```python
from build123d import *

# Parameters (mm, degrees)
SKETCH2_R           = 26.533992322
BOSS_EXTRUDE1_DEPTH = 5.7658
CHAMFER1_SIZE       = 1.27
SKETCH3_R           = 8.509
CUT_EXTRUDE1_DEPTH  = 5.7658
CHAMFER2_SIZE       = 1.016


with BuildPart() as part:
    # Sketch2 → Boss-Extrude1 (new body)
    with BuildSketch(Plane.XY):
        with Locations(Location((0, 0, 0), (0, 0, 180))):
            Circle(SKETCH2_R)
    extrude(amount=BOSS_EXTRUDE1_DEPTH)

    # Chamfer1
    chamfer1_edges = [part.edges().sort_by_distance(p)[0] for p in [
        (26.533992322, 0, 0),
        (26.533992322, 0, 5.7658),
    ]]
    chamfer(chamfer1_edges, length=CHAMFER1_SIZE)

    # Sketch3 → Cut-Extrude1 (cut)
    with BuildSketch(Plane.XY.offset(5.7658)):
        Circle(SKETCH3_R)
    extrude(amount=-CUT_EXTRUDE1_DEPTH, mode=Mode.SUBTRACT)

    # Chamfer2
    chamfer2_edges = [part.edges().sort_by_distance(p)[0] for p in [
        (-8.509, 0, 0),
        (-8.509, 0, 5.7658),
    ]]
    chamfer(chamfer2_edges, length=CHAMFER2_SIZE)


solid = part.part
```
Can you work these out from the model? Positions are in its coordinate system, mm. Give positions to 0.01 mm unless a question says otherwise; leave off trailing zeros. Write each loop counter-clockwise with the first axis right and the second up, starting at its lowest first coordinate (ties: lowest second). Pieces come first, ordered by that corner, then holes. Notation, with made-up numbers: (-3.5, 66) -> (34.5, 66) arc R27 ccw to (34.5, 104) -> close; hole circle Ø2 at (59, 35.25). An arc over 180 degrees is marked (long way). Write item = value, one per line.
(1) Suppose I cut it at C-C on z = 2.3. Write out the boundary of the cut face in (x, y), then the cut area to 3 significant figures.
Worked out:
outline = circle Ø53.07 at (0, 0); hole circle Ø17.02 at (0, 0)
area = 1,980 mm^2
(2) Suppose I cut it at A-A on y = 0. Write out the boundary of the cut face in (x, z) (3 decimals), then the cut area to 3 significant figures.
Worked out:
outline = (-26.534, 1.27) -> (-25.264, 0) -> (-9.525, 0) -> (-8.509, 1.016) -> (-8.509, 4.75) -> (-9.525, 5.766) -> (-25.264, 5.766) -> (-26.534, 4.496) -> close; (8.509, 1.016) -> (9.525, 0) -> (25.264, 0) -> (26.534, 1.27) -> (26.534, 4.496) -> (25.264, 5.766) -> (9.525, 5.766) -> (8.509, 4.75) -> close
area = 203 mm^2
(3) I need wall thicknesses on probe 1 along Y at (x, z) = (0, 2.15); probe 2 along Y at (x, z) = (3.5, 1.1); probe 3 along X at (y, z) = (6, 2.05). Which ranges of each line are inside material? Lowest first, please. Write a range as from..to.
Worked out:
probe_1 = -26.53..-8.51, 8.51..26.53
probe_2 = -26.13..-7.76, 7.76..26.13
probe_3 = -25.85..-6.03, 6.03..25.85
(4) I'm going to push flat-ended pins straight in: P1, Ø22, axis at x = 0, y = 0, coming from the -Z side; P2, Ø3, axis at x = -3, z = 4, coming from the +Y side; P3, Ø2, axis at y = -13.5, z = 0.5, coming from the -X side. Where does each tip first touch, or does it pass through?
Worked out:
P1 = 0
P2 = 26.49
P3 = -23.21
(5) Thinking about a two-plate mould opening in Y: for faces 1 (the face through (-1.108, 8.437, 2.909)), 2 (the face through (-11, 0, 5.766)), 3 (the face through (5.752, 25.903, 2.86)), which applies, released by +Y, released by -Y, zero draft, split by the parting line, or undercut?
Worked out:
face_1 = undercut
face_2 = zero draft
face_3 = split by the parting line
